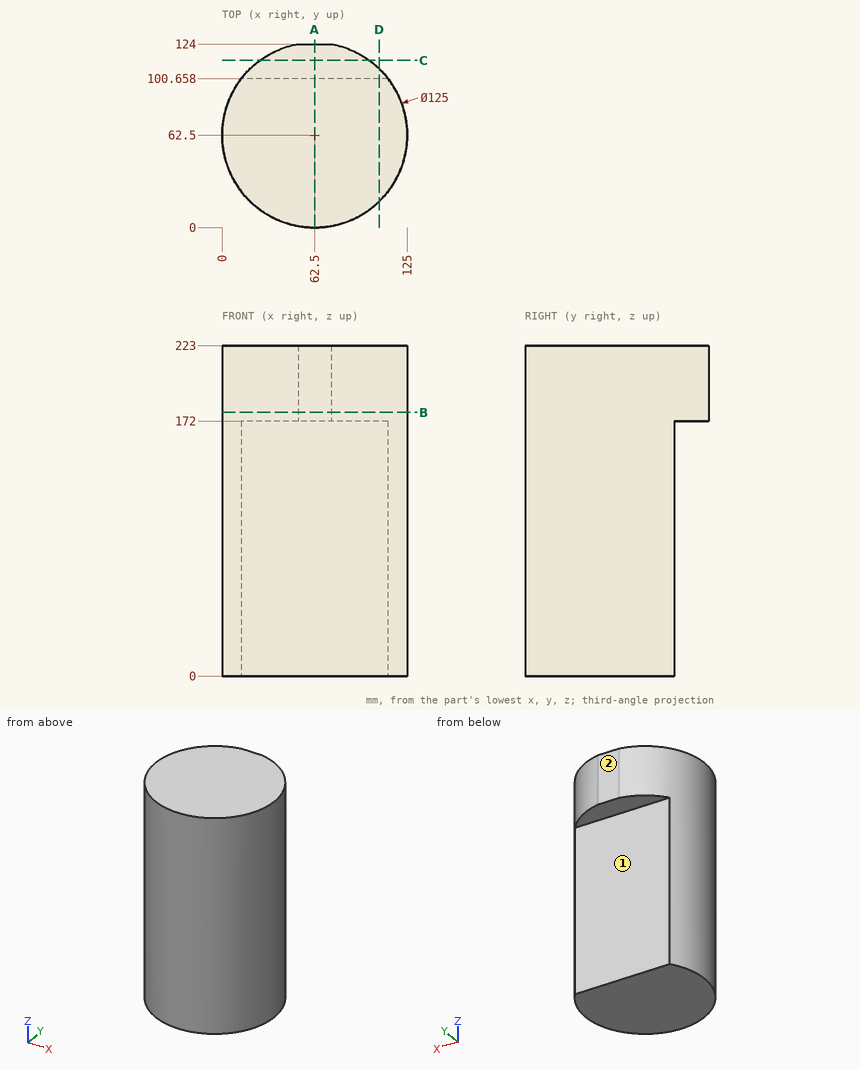
Print and shaded views of the part. All mm, measured from the part's lowest x, y and z. A direction names the side the tool comes from. Give positions to 0.01 mm unless a question says otherwise; leave off trailing zeros. Loops run counter-clockwise (first coordinate to the right, second up) from the corner with the lowest first, then second, coordinate; pieces in that order, holes last. Notation, with made-up numbers: (34, 49.25) -> (67, 49.25) arc R18 ccw to (67, 59.25) -> close; hole circle Ø5 at (45, 48.25). An arc over 180 degrees is marked (long way). Use a Markdown table: item, result.
1. Wall check: L1, parallel to Z at x = 37, y = 111.5; L2, parallel to Y at x = 47.5, z = 96.5; L3, parallel to X at y = 98, z = 95. Give the ranges that are in metal, low to high. Write a range as [from, to].
Check result:
| item | result |
|---|---|
| L1 | z = [172, 223] |
| L2 | y = [1.83, 100.66] |
| L3 | x = [11.06, 113.94] |
2. Slice it at C-C (y = 113). List the corners of the cut face in (x, z), plus the area to 3 significant figures.
Check result:
| item | result |
|---|---|
| outline | (25.68, 172) -> (99.32, 172) -> (99.32, 223) -> (25.68, 223) -> close |
| area | 3,760 mm^2 |
3. Flat gauge pins, fed straight in: pin 1 (12 mm diameter, centred on x = 18, z = 176, fed in from +Y) (1 decimal); pin 2 (4 mm diameter, centred on x = 22, z = 107.5, fed in from -Y) (1 decimal); pin 3 (6 mm diameter, centred on x = 95, y = 109, fed in from -Z). Where does each tip first touch, or does it go through?
Check result:
| item | result |
|---|---|
| pin 1 | stops at y = 111.7 |
| pin 2 | stops at y = 13.3 |
| pin 3 | stops at z = 172 |
4. Which spindle directions (+Z, -Z, +X, -X, +Y, -Y) get a long thin tool onto all of the face, cutting with end or side? Do the marked faces 1 and 2. Say none if no direction does.
Check result:
| item | result |
|---|---|
| face 1 | -Z, +X, -X, +Y |
| face 2 | +Z, -Z, +X, -X, +Y |
5. Slice it at D-D (x = 106). List the corners of the cut face in (y, z), plus the area to 3 significant figures.
Check result:
| item | result |
|---|---|
| outline | (17.62, 0) -> (100.66, 0) -> (100.66, 172) -> (107.38, 172) -> (107.38, 223) -> (17.62, 223) -> close |
| area | 18,900 mm^2 |
6. Slice it at A-A (x = 62.5). List the corners of the cut face in (y, z), plus the area to 3 significant figures.
Check result:
| item | result |
|---|---|
| outline | (0, 0) -> (100.66, 0) -> (100.66, 172) -> (124, 172) -> (124, 223) -> (0, 223) -> close |
| area | 23,600 mm^2 |
7. Slice it at B-B (z = 178). List the corners of the cut face in (x, y) (1 decimal).
Check result:
| item | result |
|---|---|
| outline | (51.4, 124) arc R62.5 ccw (long way) to (73.6, 124) -> close |
